Verification items for the finished model (mm, model axes). A direction names the side the tool comes from. Round coordinates to 2 decimals unless told otherwise and drop trailing zeros. Order: outer loops, then holes, each group sorted by start corner. A loop starts at its lowest first (then second) coordinate and runs counter-clockwise, first axis right, second up. Notation, with made-up numbers: M 56,-11 L 109,-11 A7 ccw 109,-1 Z; hole C 78.5,-4.5 d3. An arc over 180 degrees is marked long. Use one line per item in the form item = value. Start each with the question number.
Item 1: Thickness scan on probe 1 along Y at (x, z) = (0, 5.5); probe 2 along Y at (x, z) = (26, 4); probe 3 along Y at (x, z) = (23, 8). Record the ranges inside material, lowest first. Write a range as [from, to].
Item 2: Go/stop test with flat-tipped pins: pin 1 Ø2.5 at (y, z) = (24, 4) entering from -X; pin 2 Ø10 at (x, y) = (-7, -21.5) entering from -Z; pin 3 Ø2 at (y, z) = (-5, 2) entering from -X; pin 4 Ø4.5 at (y, z) = (-24, 10) entering from +X. Record where each tip stops, or that it passes through.
Item 3: Cross-section at A-A on y = 0. Enter the section's corners in (x, z), then the cut area to 3 significant figures.
Item 4: Tool access check on faces 1 (the cylindrical face through (19.31, -22.96, 6.9)), 2 (the flat face through (-25.46, 2.255, 6.902)), 3 (the flat face through (2.2, 25, 7)), 4 (the flat face through (25.336, 2.233, 6.902)), 5 (the flat face through (-10.78, 23.18, 6.9)). Record the directions out of +Z, -Z, +X, -X, +Y, -Y that give a thin tool (end or side, any length) a straight path to the whole face; none if there is none.
Item 5: Cross-section at B-B on x = 0. Enter the section's corners in (y, z), then the cut area to 3 significant figures.
Item 6: Release check for a two-part mould opening along X. For faces 6 (the cylindrical face through (-25.965, -15.027, 6.902)), 7 (the cylindrical face through (19.26, 23, 6.9)), 8 (the cylindrical face through (-14.6, 11.2, 6.9)) record: +X half, -X half, draft (parallel to the pull), parting line (faces both ways), or undercut.
Item 7: Cross-section at C-C on x = 26. Enter the section's corners in (y, z), then the cut area to 3 significant figures.
Autodesk Inventor part; units mm, degrees
ref_plane "YZ Plane" through (0, 0, 0) normal (1, 0, 0) x (0, 1, 0)
ref_plane "XZ Plane" through (0, 0, 0) normal (0, 1, 0) x (-1, 0, 0)
ref_plane "XY Plane" through (0, 0, 0) normal (0, 0, 1) x (1, 0, 0)
sketch "스케치1" plane through (0, 0, 0) normal (0, 0, 1) x (1, 0, 0)
  circle A0 centre (0, 0) radius 18.4
  arc A1 (2.2, 29.9192) -> (-2.2, 29.9192) centre (0, 0) ccw
  arc A2 (-2.2, 20.8844) -> (2.2, 20.8844) centre (0, 0) ccw
  line L0 (2.2, 29.9192) -> (-2.2, 29.9192)
  line L1 (-2.2, 29.9192) -> (-2.2, 20.8844)
  line L2 (2.2, 20.8844) -> (2.2, 29.9192)
  arc A3 (-8.1657, 28.8673) -> (-12.3003, 27.3624) centre (0, 0) ccw
  line L3 (-8.1657, 28.8673) -> (-12.3003, 27.3624)
  line L4 (-12.3003, 27.3624) -> (-9.2102, 18.8725)
  line L5 (-5.0756, 20.3774) -> (-8.1657, 28.8673)
  arc A4 (-17.5464, 24.3336) -> (-20.917, 21.5053) centre (0, 0) ccw
  line L6 (-17.5464, 24.3336) -> (-20.917, 21.5053)
  line L7 (-20.917, 21.5053) -> (-15.1096, 14.5843)
  line L8 (-11.739, 17.4125) -> (-17.5464, 24.3336)
  arc A5 (-24.8108, 16.8649) -> (-27.0108, 13.0544) centre (0, 0) ccw
  line L9 (-24.8108, 16.8649) -> (-27.0108, 13.0544)
  line L10 (-27.0108, 13.0544) -> (-19.1865, 8.537)
  line L11 (-16.9865, 12.3475) -> (-24.8108, 16.8649)
  arc A6 (-29.0827, 7.362) -> (-29.8467, 3.0288) centre (0, 0) ccw
  line L12 (-29.0827, 7.362) -> (-29.8467, 3.0288)
  line L13 (-29.8467, 3.0288) -> (-20.9492, 1.46)
  line L14 (-20.1851, 5.7931) -> (-29.0827, 7.362)
  arc A7 (-29.8467, -3.0288) -> (-29.0827, -7.362) centre (0, 0) ccw
  line L15 (-29.8467, -3.0288) -> (-29.0827, -7.362)
  line L16 (-29.0827, -7.362) -> (-20.1851, -5.7931)
  line L17 (-20.9492, -1.46) -> (-29.8467, -3.0288)
  arc A8 (-27.0108, -13.0544) -> (-24.8108, -16.8649) centre (0, 0) ccw
  line L18 (-27.0108, -13.0544) -> (-24.8108, -16.8649)
  line L19 (-24.8108, -16.8649) -> (-16.9865, -12.3475)
  line L20 (-19.1865, -8.537) -> (-27.0108, -13.0544)
  arc A9 (-20.917, -21.5053) -> (-17.5464, -24.3336) centre (0, 0) ccw
  line L21 (-20.917, -21.5053) -> (-17.5464, -24.3336)
  line L22 (-17.5464, -24.3336) -> (-11.739, -17.4125)
  line L23 (-15.1096, -14.5843) -> (-20.917, -21.5053)
  arc A10 (-12.3003, -27.3624) -> (-8.1657, -28.8673) centre (0, 0) ccw
  line L24 (-12.3003, -27.3624) -> (-8.1657, -28.8673)
  line L25 (-8.1657, -28.8673) -> (-5.0756, -20.3774)
  line L26 (-9.2102, -18.8725) -> (-12.3003, -27.3624)
  arc A11 (-2.2, -29.9192) -> (2.2, -29.9192) centre (0, 0) ccw
  line L27 (-2.2, -29.9192) -> (2.2, -29.9192)
  line L28 (2.2, -29.9192) -> (2.2, -20.8844)
  line L29 (-2.2, -20.8844) -> (-2.2, -29.9192)
  arc A12 (8.1657, -28.8673) -> (12.3003, -27.3624) centre (0, 0) ccw
  line L30 (8.1657, -28.8673) -> (12.3003, -27.3624)
  line L31 (12.3003, -27.3624) -> (9.2102, -18.8725)
  line L32 (5.0756, -20.3774) -> (8.1657, -28.8673)
  arc A13 (17.5464, -24.3336) -> (20.917, -21.5053) centre (0, 0) ccw
  line L33 (17.5464, -24.3336) -> (20.917, -21.5053)
  line L34 (20.917, -21.5053) -> (15.1096, -14.5843)
  line L35 (11.739, -17.4125) -> (17.5464, -24.3336)
  arc A14 (24.8108, -16.8649) -> (27.0108, -13.0544) centre (0, 0) ccw
  line L36 (24.8108, -16.8649) -> (27.0108, -13.0544)
  line L37 (27.0108, -13.0544) -> (19.1865, -8.537)
  line L38 (16.9865, -12.3475) -> (24.8108, -16.8649)
  arc A15 (29.0827, -7.362) -> (29.8467, -3.0288) centre (0, 0) ccw
  line L39 (29.0827, -7.362) -> (29.8467, -3.0288)
  line L40 (29.8467, -3.0288) -> (20.9492, -1.46)
  line L41 (20.1851, -5.7931) -> (29.0827, -7.362)
  arc A16 (29.8467, 3.0288) -> (29.0827, 7.362) centre (0, 0) ccw
  line L42 (29.8467, 3.0288) -> (29.0827, 7.362)
  line L43 (29.0827, 7.362) -> (20.1851, 5.7931)
  line L44 (20.9492, 1.46) -> (29.8467, 3.0288)
  arc A17 (27.0108, 13.0544) -> (24.8108, 16.8649) centre (0, 0) ccw
  line L45 (27.0108, 13.0544) -> (24.8108, 16.8649)
  line L46 (24.8108, 16.8649) -> (16.9865, 12.3475)
  line L47 (19.1865, 8.537) -> (27.0108, 13.0544)
  arc A18 (20.917, 21.5053) -> (17.5464, 24.3336) centre (0, 0) ccw
  line L48 (20.917, 21.5053) -> (17.5464, 24.3336)
  line L49 (17.5464, 24.3336) -> (11.739, 17.4125)
  line L50 (15.1096, 14.5843) -> (20.917, 21.5053)
  arc A19 (12.3003, 27.3624) -> (8.1657, 28.8673) centre (0, 0) ccw
  line L51 (12.3003, 27.3624) -> (8.1657, 28.8673)
  line L52 (8.1657, 28.8673) -> (5.0756, 20.3774)
  line L53 (9.2102, 18.8725) -> (12.3003, 27.3624)
  dimension "d6" = 360
extrude "돌출1" add sketch "스케치1" along normal blind 14
properties part number "Dummy_Stator"
Output values:
q1.probe_1 = [-30, -18.4], [18.4, 30]
q1.probe_2 = [-14.97, -12.47], [-6.82, -2.35], [2.35, 6.82], [12.47, 14.97]
q1.probe_3 = [-15.82, -10.74], [-6.29, -1.82], [1.82, 6.29], [10.74, 15.82]
q2.pin_1 = -19.56
q2.pin_2 = 0
q2.pin_3 = -29.73
q2.pin_4 = 20.66
q3.outline = M -21,0 L -18.4,0 L -18.4,14 L -21,14 Z; M 18.4,0 L 21,0 L 21,14 L 18.4,14 Z
q3.area = 72.8 mm2
q4.face_1 = +Z, -Z, +X, -Y
q4.face_2 = +Z, -Z, -X
q4.face_3 = +Z, -Z, +Y
q4.face_4 = +Z, -Z, +X
q4.face_5 = +Z, -Z
q5.outline = M -30,0 L -18.4,0 L -18.4,14 L -30,14 Z; M 18.4,0 L 30,0 L 30,14 L 18.4,14 Z
q5.area = 325 mm2
q6.face_6 = -X half
q6.face_7 = +X half
q6.face_8 = undercut
q7.outline = M -14.97,0 L -12.47,0 L -12.47,14 L -14.97,14 Z; M -6.82,0 L -2.35,0 L -2.35,14 L -6.82,14 Z; M 2.35,0 L 6.82,0 L 6.82,14 L 2.35,14 Z; M 12.47,0 L 14.97,0 L 14.97,14 L 12.47,14 Z
q7.area = 195 mm2
